Job drawing, mm, ordinate dimensions from the low corner. One solid piece. Round coordinates to 2 decimals unless told otherwise and drop trailing zeros. Write each loop counter-clockwise with the first axis right and the second up, starting at its lowest first coordinate (ties: lowest second). Pieces come first, ordered by that corner, then holes.
1) Saw through at A-A on z = 53.5. Write the cut outline in (x, y).
2) Drill centre lines: L1, parallel to Y at x = 10, z = 3; L2, parallel to X at y = 15.25, z = 24.5; L3, parallel to X at y = 16.75, z = 38. Where is each one in solid material? Low to high.
3) Saw through at C-C on z = 22. Write the cut outline in (x, y).
4) Flat gauge pins, fed straight in: pin 1 (5 mm diameter, centred on x = 5.5, y = 3.5, fed in from -Z); pin 2 (3 mm diameter, centred on x = 10, y = 10, fed in from +Z); pin 3 (1.5 mm diameter, centred on y = 3, z = 27.5, fed in from -X). Where does each tip first touch, or does it go through?
5) Saw through at B-B on y = 10. Write the cut outline in (x, z), and give its area (4 significant figures).
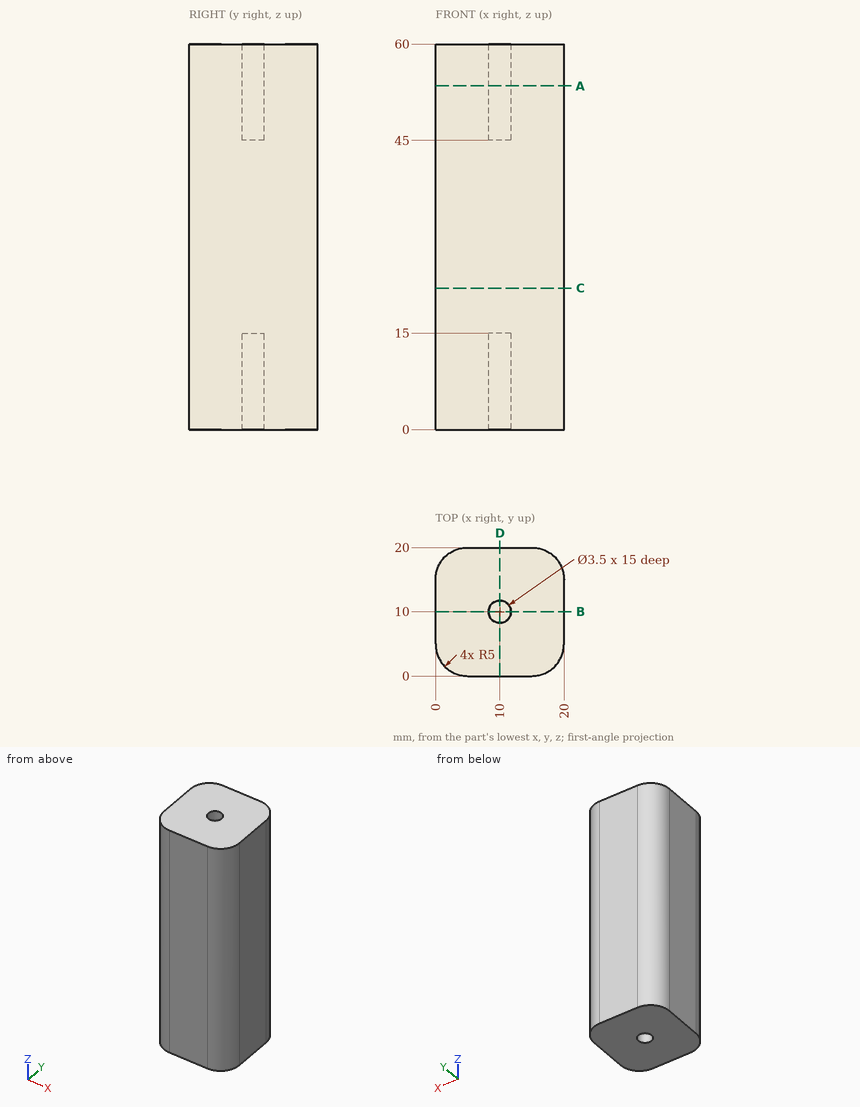
Completed:
1. outline: (0, 5) arc R5 ccw to (5, 0) - (15, 0) arc R5 ccw to (20, 5) - (20, 15) arc R5 ccw to (15, 20) - (5, 20) arc R5 ccw to (0, 15) - close; hole circle Ø3.5 at (10, 10)
2. L1: y = 0 to 8.25, 11.75 to 20
2. L2: x = 0.01 to 19.99
2. L3: x = 0.32 to 19.68
3. outline: (0, 5) arc R5 ccw to (5, 0) - (15, 0) arc R5 ccw to (20, 5) - (20, 15) arc R5 ccw to (15, 20) - (5, 20) arc R5 ccw to (0, 15) - close
4. pin 1: stops at z = 0
4. pin 2: stops at z = 45
4. pin 3: stops at x = 0.16
5. outline: (0, 0) - (8.25, 0) - (8.25, 15) - (11.75, 15) - (11.75, 0) - (20, 0) - (20, 60) - (11.75, 60) - (11.75, 45) - (8.25, 45) - (8.25, 60) - (0, 60) - close
5. area: 1,095 mm2
